Autodesk Inventor part; units mm, degrees
ref_plane "YZ Plane" through (0, 0, 0) normal (1, 0, 0) x (0, 1, 0)
ref_plane "XZ Plane" through (0, 0, 0) normal (0, 1, 0) x (-1, 0, 0)
ref_plane "XY Plane" through (0, 0, 0) normal (0, 0, 1) x (1, 0, 0)
sketch "Sketch1" plane through (0, 0, 0) normal (0, 0, 1) x (1, 0, 0)
  line L0 (-15, 2) -> (15, 2)
  line L1 (15, 2) -> (15, -2)
  line L2 (15, -2) -> (-15, -2)
  line L3 (-15, -2) -> (-15, 2)
  line L4 (-15, 2) -> (15, -2) construction
  line L5 (15, 2) -> (-15, -2) construction
  point P0 (0, 0)
  dimension "d0" = 30
  dimension "d1" = 4
extrude "Extrusion1" add sketch "Sketch1" along normal blind 8
sketch "Sketch2" plane through (0, 0, 8) normal (0, 0, 1) x (1, 0, 0)
  point P0 (0, 0)
ref_plane "Work Plane2" through (0, -28.25, 4) normal (0, 0, 1) x (1, 0, 0)
sketch "Sketch4" plane through (0, -28.25, 4) normal (0, 0, 1) x (1, 0, 0)
  line L0 (-66.5, 32.5) -> (66.5, 32.5)
  line L1 (66.5, 32.5) -> (66.5, -32.5)
  line L2 (66.5, -32.5) -> (-66.5, -32.5)
  line L3 (-66.5, -32.5) -> (-66.5, 32.5)
  line L4 (-66.5, 32.5) -> (66.5, -32.5) construction
  line L5 (66.5, 32.5) -> (-66.5, -32.5) construction
  line L6 (15, 26.25) -> (15, 30.25)
  point P0 (0, 28.25)
  point P1 (0, 0)
  dimension "d4" = 133
  dimension "d5" = 65
extrude "Extrusion2" add sketch "Sketch4" along normal blind 2
properties part number "Top"
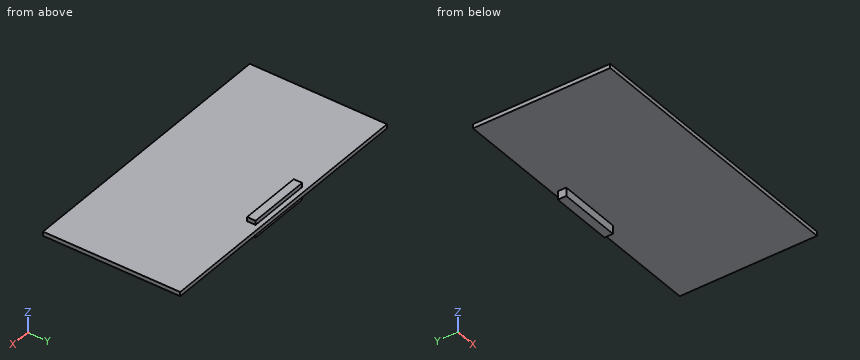
Input: part model. Units: mm. Frame: model coordinates. Coordinates: 2 decimals unless noted, no trailing zeros. Write each loop counter-clockwise with the first axis right and the second up, starting at its lowest first coordinate (ties: lowest second). Pieces come first, ordered by that corner, then holes. Notation, with made-up numbers: M -8,-29 L 33,-29 A17 ccw 33,-10 Z; hole C -24.75,43.25 d1. An arc over 180 degrees is marked long. Answer as a JSON object with one key per item and string values. Group by question number.
(1) Contact query for flat-ended pins moving along their axis: P1, Ø4, axis at x = -36, y = -51.5, coming from the -Z side; P2, Ø3, axis at x = 2, z = 3, coming from the +Y side; P3, Ø1, axis at x = -4, z = 7.5, coming from the -Y side; P4, Ø1.6, axis at x = 1, z = 7, coming from the +Y side. Output: stop coordinate, or through.
(2) Section C-C on y = -33. Output: boundary loops of the cut face in (x, z).
(3) Ray query, line 1 along Z through (x, y) = (-23, -25). Return the intervals inside material, ascending. Write a range as [from, to].
(4) Section B-B on z = 2. Output: boundary loops of the cut face in (x, y).
(5) Section A-A on x = 3. Output: boundary loops of the cut face in (y, z), plus the area to 3 significant figures.
Result set:
{
 "1": {"P1": "stops at z = 4", "P2": "stops at y = 4.25", "P3": "stops at y = -2", "P4": "stops at y = 2"},
 "2": {"outline": "M -66.5,4 L 66.5,4 L 66.5,6 L -66.5,6 Z"},
 "3": {"line 1": "z = [4, 6]"},
 "4": {"outline": "M -15,-2 L 15,-2 L 15,2 L -15,2 Z"},
 "5": {"outline": "M -60.75,4 L -2,4 L -2,0 L 2,0 L 2,4 L 4.25,4 L 4.25,6 L 2,6 L 2,8 L -2,8 L -2,6 L -60.75,6 Z", "area": "154 mm2"}
}
